```python
from build123d import *

# Parameters (mm, degrees)
SKETCH_W           = 4.4
SKETCH_H           = 4.4
PAD_DEPTH          = 2.8
SKETCH001_R        = 3.7
PAD001_DEPTH       = 0.6
SKETCH002_W        = 1.6
SKETCH002_H        = 3
POCKET_DEPTH       = 22.267564
POLARPATTERN_COUNT = 4
SKETCH003_W        = 3.8
SKETCH003_H        = 3.8
POCKET001_DEPTH    = 1.9


with BuildPart() as part:
    # Sketch → Pad (new body)
    with BuildSketch(Plane.XY):
        Rectangle(SKETCH_W, SKETCH_H)
    extrude(amount=PAD_DEPTH)

    # Sketch001 → Pad001 (join)
    with BuildSketch(Plane.XY):
        Circle(SKETCH001_R)
    extrude(amount=PAD001_DEPTH)

    # Sketch002 (on DatumPlane) → Pocket (cut, through all)
    with BuildSketch(Plane.XY.offset(0.6)):
        with Locations((0, 3.7)):
            Rectangle(SKETCH002_W, SKETCH002_H)
    pocket = extrude(amount=-POCKET_DEPTH, mode=Mode.SUBTRACT)

    # PolarPattern: Pocket ×4 about axis
    polarpattern_axis = Axis((0, 0, 0.6), (0, 0, 1))
    for i in range(1, POLARPATTERN_COUNT):
        add(pocket.rotate(polarpattern_axis, i * 360 / POLARPATTERN_COUNT), mode=Mode.SUBTRACT)

    # Sketch003 (on DatumPlane) → Pocket001 (cut)
    with BuildSketch(Plane(origin=(0, 0, 0), x_dir=(1, 0, 0), z_dir=(0, 0, -1))):
        Rectangle(SKETCH003_W, SKETCH003_H)
    extrude(amount=-POCKET001_DEPTH, mode=Mode.SUBTRACT)


solid = part.part
```
Can you work these out from the model? Positions are in its coordinate system, mm. A direction names the side the tool comes from. Coordinates: 2 decimals unless noted, no trailing zeros. Loops run counter-clockwise (first coordinate to the right, second up) from the corner with the lowest first, then second, coordinate; pieces in that order, holes last.
Item 1: If we mould it in two halves opening along X, with no side actions, what happens to faces 3 (the face through (-2.637, -2.595, 0.296)), 4 (the face through (1.9, 0, 1)), 5 (the face through (2.637, 2.595, 0.296)), 6 (the face through (-2.5, -2.2, 0.6))? For each: released by +X, released by -X, zero draft, split by the parting line, or undercut.
Answers below:
face 3: released by -X
face 4: undercut
face 5: released by +X
face 6: zero draft
Item 2: Suppose I cut it at B-B (z = 0.25). Please give me the cut outline in (x, y), then the cut area to 3 significant figures.
Answers below:
outline: (-3.61, -0.8) arc R3.7 ccw to (-0.8, -3.61) - (-0.8, -2.2) - (0.8, -2.2) - (0.8, -3.61) arc R3.7 ccw to (3.61, -0.8) - (2.2, -0.8) - (2.2, 0.8) - (3.61, 0.8) arc R3.7 ccw to (0.8, 3.61) - (0.8, 2.2) - (-0.8, 2.2) - (-0.8, 3.61) arc R3.7 ccw to (-3.61, 0.8) - (-2.2, 0.8) - (-2.2, -0.8) - close; hole (-1.9, -1.9) - (1.9, -1.9) - (1.9, 1.9) - (-1.9, 1.9) - close
area: 19.2 mm2
Item 3: Suppose I cut it at D-D (x = 3). Please give me the cut outline in (y, z), then the cut area to 3 significant figures.
Answers below:
outline: (-2.17, 0) - (-0.8, 0) - (-0.8, 0.6) - (-2.17, 0.6) - close; (0.8, 0) - (2.17, 0) - (2.17, 0.6) - (0.8, 0.6) - close
area: 1.64 mm2
Item 4: Which directions (+Z, -Z, +X, -X, +Y, -Y) give clear straight access to the entire face, cutting with the end or side of a thin tool? Please do faces 1 (the face through (0, 0, 1.9)), 2 (the face through (-2.595, 2.637, 0.296)).
Answers below:
face 1: -Z
face 2: +Z, -Z, -X, +Y
Item 5: Suppose I cut it at A-A (x = 0.5). Please give me the cut outline in (y, z).
Answers below:
outline: (-2.2, 0) - (-1.9, 0) - (-1.9, 1.9) - (1.9, 1.9) - (1.9, 0) - (2.2, 0) - (2.2, 2.8) - (-2.2, 2.8) - close
Item 6: I'm going to push flat-ended pins straight in: pin 1 (1.4 mm diameter, centred on x = 0.5, z = 1.5, fed in from -Y); pin 2 (0.7 mm diameter, centred on y = 3, z = 0.5, fed in from +X); pin 3 (0.7 mm diameter, centred on x = -3, z = 0.5, fed in from -Y). Where does each tip first touch, or does it pass through?
Answers below:
pin 1: stops at y = -2.2
pin 2: stops at x = 2.58
pin 3: stops at y = -2.58
Item 7: Please list where these lines run through material, in increasing order: L1, parallel to Y at x = 0.75, z = 0.85; L2, parallel to Z at x = -2.25, y = 2.5.
Answers below:
L1: y = -2.2 to -1.9, 1.9 to 2.2
L2: z = 0 to 0.6
